```python
from build123d import *

# Parameters (mm, degrees)
BOSS_EXTRUDE1_DEPTH  = 15.875
SKETCH2_R            = 1.5875
MOUNTING_HOLES_DEPTH = 52.199274653
SKETCH3_W            = 13.2
SKETCH3_H            = 19.2
CUT_EXTRUDE2_DEPTH   = 55.113625512
SKETCH4_W            = 18.28
SKETCH4_H            = 24.28
SKETCH4_W_2          = 13.2
SKETCH4_H_2          = 19.2
CUT_EXTRUDE3_DEPTH   = 1.905
FILLET2_R            = 0.635
FILLET3_R            = 0.635
BOSS_EXTRUDE3_DEPTH  = 2.54
FILLET4_R            = 0.635
FILLET5_R            = 1.905


with BuildPart() as part:
    # Sketch1 → Boss-Extrude1 (new, symmetric)
    with BuildSketch(Plane(origin=(0, 0, 0), x_dir=(1, 0, 0), z_dir=(0, 1, 0))):
        Polygon((0, 0), (0, 12.7), (3.81, 12.7), (3.81, 2.921), (50.8, 2.921), (50.8, 0), align=None)
    extrude(amount=BOSS_EXTRUDE1_DEPTH, both=True)

    # Sketch2 → Mounting_Holes (cut, through all)
    with BuildSketch(Plane(origin=(3.81, 0, 0), x_dir=(0, 0, -1), z_dir=(1, 0, 0))):
        with Locations((6.35, 9.525)):
            Circle(SKETCH2_R)
        with Locations((6.35, -9.525)):
            Circle(SKETCH2_R)
    extrude(amount=-MOUNTING_HOLES_DEPTH, mode=Mode.SUBTRACT)

    # Sketch3 → Cut-Extrude2 (cut, through all)
    with BuildSketch(Plane(origin=(0, 0, -2.921), x_dir=(-1, 0, 0), z_dir=(0, 0, -1))):
        with Locations((-37.715, 0)):
            Rectangle(SKETCH3_W, SKETCH3_H)
        with Locations((-16.895, 0)):
            Rectangle(SKETCH3_W, SKETCH3_H)
    extrude(amount=-CUT_EXTRUDE2_DEPTH, mode=Mode.SUBTRACT)

    # Sketch4 → Cut-Extrude3 (cut)
    # profile 1 of 2: a face of its own
    with BuildSketch(Plane(origin=(0, 0, -2.921), x_dir=(-1, 0, 0), z_dir=(0, 0, -1))):
        with Locations((-37.715, 0)):
            Rectangle(SKETCH4_W, SKETCH4_H)
        with Locations((-37.715, 0)):
            Rectangle(SKETCH4_W_2, SKETCH4_H_2, mode=Mode.SUBTRACT)
    # profile 2 of 2: a face of its own
    with BuildSketch(Plane(origin=(0, 0, -2.921), x_dir=(-1, 0, 0), z_dir=(0, 0, -1))):
        with Locations((-16.895, 0)):
            Rectangle(SKETCH4_W, SKETCH4_H)
        with Locations((-16.895, 0)):
            Rectangle(SKETCH4_W_2, SKETCH4_H_2, mode=Mode.SUBTRACT)
    extrude(amount=-CUT_EXTRUDE3_DEPTH, mode=Mode.SUBTRACT)

    # Fillet2
    fillet2_edges = [part.edges().sort_by_distance(p)[0] for p in [
        (3.81, 0, -2.921),
        (23.495, -9.6, -0.508),
        (23.495, 9.6, -0.508),
        (10.295, 9.6, -0.508),
        (10.295, -9.6, -0.508),
        (44.315, 9.6, -0.508),
        (31.115, 9.6, -0.508),
        (31.115, -9.6, -0.508),
        (44.315, -9.6, -0.508),
    ]]
    fillet(fillet2_edges, radius=FILLET2_R)

    # Fillet3
    fillet3_edges = [part.edges().sort_by_distance(p)[0] for p in [
        (28.575, 0, -1.016),
        (28.575, 12.14, -1.9685),
        (37.715, -12.14, -1.016),
        (46.855, 0, -1.016),
        (46.855, -12.14, -1.9685),
        (37.715, 12.14, -1.016),
        (46.855, 12.14, -1.9685),
        (7.755, 0, -1.016),
        (7.755, 12.14, -1.9685),
        (16.895, -12.14, -1.016),
        (7.755, -12.14, -1.9685),
        (26.035, 0, -1.016),
        (26.035, -12.14, -1.9685),
        (16.895, 12.14, -1.016),
        (26.035, 12.14, -1.9685),
    ]]
    fillet(fillet3_edges, radius=FILLET3_R)

    # Sketch5 → Boss-Extrude3 (add)
    with BuildSketch(Plane.XZ.offset(15.875)):
        Polygon((50.8, 0), (50.8, -22.86), (41.275, -22.86), (41.275, -20.32), (45.085, -20.32), (45.085, -16.51), (32.385, -16.51), (32.385, -20.32), (36.195, -20.32), (36.195, -22.86), (19.05, -22.86), (19.05, -20.32), (22.86, -20.32), (22.86, -16.51), (10.16, -16.51), (10.16, -20.32), (13.97, -20.32), (13.97, -22.86), (0, -22.86), (0, 0), align=None)
    extrude(amount=-BOSS_EXTRUDE3_DEPTH)

    # Fillet4
    fillet4_edges = [part.edges().sort_by_distance(p)[0] for p in [
        (45.085, -14.605, -20.32),
        (45.085, -14.605, -16.51),
        (32.385, -14.605, -16.51),
        (32.385, -14.605, -20.32),
        (22.86, -14.605, -20.32),
        (22.86, -14.605, -16.51),
        (10.16, -14.605, -16.51),
        (10.16, -14.605, -20.32),
    ]]
    fillet(fillet4_edges, radius=FILLET4_R)

    # Fillet5
    fillet5_edges = [part.edges().sort_by_distance(p)[0] for p in [
        (0, 15.875, -6.35),
        (0, -15.875, -11.43),
        (50.8, -15.875, -11.43),
        (50.8, 15.875, -1.4605),
    ]]
    fillet(fillet5_edges, radius=FILLET5_R)


solid = part.part
```
Can you work these out from the model? Positions are in its coordinate system, mm. A direction names the side the tool comes from. Round coordinates to 2 decimals unless told otherwise and drop trailing zeros. Loops run counter-clockwise (first coordinate to the right, second up) from the corner with the lowest first, then second, coordinate; pieces in that order, holes last. Notation, with made-up numbers: M 67.25,0 L 115.25,0 A27 cw 115.25,35 Z; hole C 24,-9.5 d1. An arc over 180 degrees is marked long. Answer in a Markdown table with one row per item.
1. If we section it at D-D, the plane z = -9.25: Please give me the cut outline in (x, y) (3 decimals), plus the area to 3 significant figures.
Established:
| item | result |
|---|---|
| outline | M 0,-13.97 A1.905 ccw 1.905,-15.875 L 48.895,-15.875 A1.905 ccw 50.8,-13.97 L 50.8,-13.335 L 3.81,-13.335 L 3.81,15.875 L 1.905,15.875 A1.905 ccw 0,13.97 Z |
| area | 238 mm² |
2. On a 3-axis mill with a long thin cutter (end or side, diameter ignored), from which of +Z, -Z, +X, -X, +Y, -Y can I reach the whole of each face in a straight line? I mean faces 1 (the face through (17, -15, -16.51)), 2 (the face through (36.195, -15, -22)), 3 (the face through (23.495, -0.1, -0.5)), 4 (the face through (17, 12.14, -2)), 5 (the face through (50.26, 15.3, -1.44)). Say none if no direction works.
Established:
| item | result |
|---|---|
| face 1 | +Y, -Y |
| face 2 | -Z, +Y, -Y |
| face 3 | +Z, -Z |
| face 4 | -Z |
| face 5 | +Z, -Z, +X, +Y |
3. If we section it at A-A, the plane y = 4: Please give me the cut outline in (x, z) (3 decimals), plus the area to 3 significant figures.
Established:
| item | result |
|---|---|
| outline | M 0,-12.7 L 3.81,-12.7 L 3.81,-3.556 A0.635 cw 4.445,-2.921 L 7.755,-2.921 L 7.755,-1.651 A0.635 cw 8.39,-1.016 L 10.295,-1.016 L 10.295,0 L 0,0 Z; M 23.495,-1.016 L 25.4,-1.016 A0.635 cw 26.035,-1.651 L 26.035,-2.921 L 28.575,-2.921 L 28.575,-1.651 A0.635 cw 29.21,-1.016 L 31.115,-1.016 L 31.115,0 L 23.495,0 Z; M 44.315,-1.016 L 46.22,-1.016 A0.635 cw 46.855,-1.651 L 46.855,-2.921 L 50.8,-2.921 L 50.8,0 L 44.315,0 Z |
| area | 89.6 mm² |
4. If we section it at B-B, the plane x = 16.5: Please give me the cut outline in (y, z) (3 decimals), plus the area to 3 significant figures.
Established:
| item | result |
|---|---|
| outline | M -15.875,-16.51 L -13.335,-16.51 L -13.335,-2.921 L -12.14,-2.921 L -12.14,-1.651 A0.635 cw -11.505,-1.016 L -9.6,-1.016 L -9.6,0 L -15.875,0 Z; M 9.6,-1.016 L 11.505,-1.016 A0.635 cw 12.14,-1.651 L 12.14,-2.921 L 15.875,-2.921 L 15.875,0 L 9.6,0 Z |
| area | 61.7 mm² |
5. If we section it at C-C, the plane z = -6.35: Please give me the cut outline in (x, y) (1 decimal).
Established:
| item | result |
|---|---|
| outline | M 0,-14 A1.9 ccw 1.9,-15.9 L 48.9,-15.9 A1.9 ccw 50.8,-14 L 50.8,-13.3 L 3.8,-13.3 L 3.8,-11.1 L 0,-11.1 Z; M 0,-7.9 L 3.8,-7.9 L 3.8,7.9 L 0,7.9 Z; M 0,11.1 L 3.8,11.1 L 3.8,15.9 L 1.9,15.9 A1.9 ccw 0,14 Z |
6. I'm going to push flat-ended pins straight in: pin 1 Ø0.8 at (y, z) = (-15, -18) entering from -X; pin 2 Ø2.5 at (y, z) = (-4.5, -8.5) entering from +X; pin 3 Ø12 at (x, z) = (30.5, -13) entering from +Y (3 decimals). Where does each tip first touch, or does it pass through?
Established:
| item | result |
|---|---|
| pin 1 | x = 0.11 |
| pin 2 | x = 3.81 |
| pin 3 | y = -13.335 |
7. Thinking about a two-plate mould opening in X: for faces 6 (the face through (0.54, 15.3, -6.44)), 7 (the face through (28.575, 0, -2)), 8 (the face through (2, 1, -12.7)), which applies, pulls with the +X half, pulls with the -X half, needs draft (parallel to the pull), parting line crosses it, or undercut?
Established:
| item | result |
|---|---|
| face 6 | pulls with the -X half |
| face 7 | undercut |
| face 8 | needs draft |
8. Please list where these lines run through material, in increasing order: line 1 (Y direction, x = 1.85, z = -6.35); line 2 (Y direction, x = 1.3, z = -6.35); line 3 (Z direction, x = 7, y = 12). Write a range as from..to.
Established:
| item | result |
|---|---|
| line 1 | -15.87..-11.11, -7.94..7.94, 11.11..15.87 |
| line 2 | -15.78..-11.11, -7.94..7.94, 11.11..15.78 |
| line 3 | -2.92..0 |
